Autodesk Inventor part; units mm, degrees
ref_plane "YZ Plane" through (0, 0, 0) normal (1, 0, 0) x (0, 1, 0)
ref_plane "XZ Plane" through (0, 0, 0) normal (0, 1, 0) x (-1, 0, 0)
ref_plane "XY Plane" through (0, 0, 0) normal (0, 0, 1) x (1, 0, 0)
sketch "Sketch1" plane through (0, 0, 0) normal (0, 1, 0) x (-1, 0, 0)
  circle A0 centre (0, 0) radius 3.81
  circle A1 centre (0, 0) radius 16.51
  line L0 (-7.4994, -5) -> (-1.1494, -5)
  line L1 (-1.1494, -5) -> (-1.1494, -11.35)
  line L2 (-1.1494, -11.35) -> (-7.4994, -11.35)
  line L3 (-7.4994, -11.35) -> (-7.4994, -5)
  line L4 (-7.4994, 5) -> (-1.1494, 5)
  line L5 (-1.1494, 5) -> (-1.1494, 11.35)
  line L6 (-1.1494, 11.35) -> (-7.4994, 11.35)
  line L7 (-7.4994, 11.35) -> (-7.4994, 5)
  circle A2 centre (-4.3244, -7.3812) radius 1.7526
  circle A3 centre (-4.3244, 7.3812) radius 1.7526
  line L8 (0, 0) -> (-10.16, 0)
  line L9 (0, 0) -> (10.16, 0)
  circle A4 centre (-10.16, 0) radius 1.7526
  circle A5 centre (10.16, 0) radius 1.7526
  line L10 (-4.3244, -8.175) -> (-10.16, 0)
  line L11 (-10.16, 0) -> (-4.3244, 8.175)
  line L12 (0, 0) -> (-7.2422, 4.0875)
  line L13 (0, 0) -> (-7.2422, -4.0875)
  line L14 (-7.2422, -4.0875) -> (-14.378, -8.115)
  line L15 (-7.2422, 4.0875) -> (-14.378, 8.115)
  line L16 (0, 0) -> (11.6743, -11.6743)
  line L17 (0, 0) -> (16.51, 0) construction
  line L18 (0, 0) -> (11.6743, 11.6743)
  line L19 (0, 0) -> (16.51, 0) construction
  line L20 (0, 0) -> (16.51, -6.8387)
  line L21 (0, 0) -> (17.8703, 0) construction
  line L22 (1.062, 0) -> (16.6655, -6.4632)
  line L23 (0.7509, -0.7509) -> (16.3545, -7.2141)
  point P0 (-3.318, 1.8727)
  point P1 (2.6941, 2.6941)
  point P2 (2.6941, -2.6941)
  point P3 (-3.318, -1.8727)
  point P4 (3.3444, -1.8252)
  point P5 (15.0931, -6.6917)
  point P6 (15.4042, -5.9407)
  point P7 (3.6554, -1.0742)
  dimension "d0" = 7.62
  dimension "d1" = 33.02
  dimension "d2" = 6.35
  dimension "d3" = 6.35
  dimension "d4" = 6.35
  dimension "d5" = 6.35
  dimension "d6" = 3.5052
  dimension "d7" = 3.5052
  dimension "d8" = 10.16
  dimension "d9" = 10.16
  dimension "d10" = 3.5052
  dimension "d11" = 3.5052
  dimension "d12" = 45
  dimension "d13" = 45
  dimension "d25" = 22.5
  dimension "d26" = 0.4064
  dimension "d27" = 0.4064
extrude "Extrusion1" add sketch "Sketch1" along normal blind 7.5184 contours A0 L18 A1 L22 | A5 | A3 | L4 L7 L6 L5 | A0 L12 L15 A1 L18 | L22 A1 L20 A0 | A0 L8 A4 L11 L12 | L20 A1 L23 A0 | A0 L13 L10 A4 L8 | L11 A4 L10 L14 A1 L15 | A2 | L0 L1 L2 L3 | A0 L16 A1 L14 L13 | L23 A1 L16 A0 | A4 L10 L8 | L8 L11 A4 | L11 L10 A4
extrude "Extrusion2" cut sketch "Sketch1" along normal blind 6.2992 contours A3 | L4 L7 L6 L5 | A0 L12 L15 A1 L18 | A2 | L0 L1 L2 L3 | A0 L16 A1 L14 L13
hole "Hole1" at (-10.16, 0, 0) at (10.16, 0, 0) at (4.3244, 0, -7.3812) at (4.3244, 0, 7.3812) direction (0, 1, 0) diameter 3.81 end through all
extrude "Extrusion3" cut sketch "Sketch1" along normal blind 7.5184 contours L22 A1 L20 A0 | L20 A1 L23 A0
properties part number "tab4"
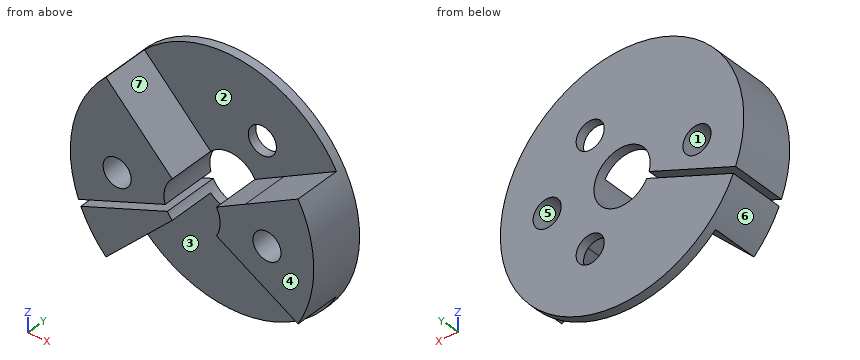
Design review of the part built by this model. Coordinates are the model's own, in mm. Face numbers are marked on the shaded views. A direction names the side the tool comes from. Give positions to 0.01 mm unless a question says otherwise; leave off trailing zeros. Order: outer loops, then holes, each group sorted by start corner. A loop starts at its lowest first (then second) coordinate and runs counter-clockwise, first axis right, second up. Notation, with made-up numbers: (6.25, 3.25) -> (43.25, 3.25) arc R17 ccw to (43.25, 18.25) -> close; hole circle Ø2 at (59.25, 54.5). An arc over 180 degrees is marked (long way). Write each question's results on one line, items separated by ' | '. Start each with the question number.
Q1. Wall thickness on L1, parallel to X at y = 5, z = 0 (3 decimals); L2, parallel to X at y = 3, z = -3.5; L3, parallel to Z at x = -11, y = 5: over which ranges is each line inside the solid? List them lowest first. Write a range as from..to.
Q2. Machinability: for the marked faces 1, 2 and 3, which of the approach directions +Z, -Z, +X, -X, +Y, -Y give a long, thin tool a straight path to every point of the face, cutting with its end or side? Answer none if there is none.
Q3. Add section C-C on z = 0. Give the boundary of the cut face in (x, y) (3 decimals), and give its area (3 significant figures).
Q4. For pin 1 (3 mm diameter, centred on x = 10.16, z = 0, fed in from -Y); pin 2 (1.5 mm diameter, centred on x = 8, y = 1, fed in from -Z); pin 3 (7.5 mm diameter, centred on x = 4, z = 12, fed in from -Y); pin 4 (6 mm diameter, centred on x = 11.5, z = 7, fed in from -Y), all flat-tipped, find the tip position at first contact; note any pin that passes through.
Q5. Mouldability with a two-part tool opening along X and no side actions: class the marked faces 4, 5, 6 and 7 as +X half, -X half, draft (parallel to the pull), parting line (faces both ways), or undercut.
Q6. Add section D-D on x = -11. Give the boundary of the cut face in (y, z).
Q7. Add section A-A on y = 3.25. Give the boundary of the cut face in (x, z) (1 decimal), and give its area (3 significant figures).
Q8. Add section B-B on x = 0. Give the boundary of the cut face in (y, z), and give its area (3 significant figures).
Found:
1) L1: x = -16.51..-12.065, -8.255..-3.81, 3.81..8.255, 12.065..16.51 | L2: x = -16.13..-9.51, -7.39..-3.5, 6.2..16.13 | L3: z = -11..-5, -4.12..-1.71, 1.71..11
2) face 1: +Y, -Y | face 2: +Z, -Y | face 3: -Z, -Y
3) outline: (-16.51, 0) -> (-12.065, 0) -> (-12.065, 7.518) -> (-16.51, 7.518) -> close; (-8.255, 0) -> (-3.81, 0) -> (-3.81, 7.518) -> (-8.255, 7.518) -> close; (3.81, 0) -> (8.255, 0) -> (8.255, 7.518) -> (3.81, 7.518) -> close; (12.065, 0) -> (16.51, 0) -> (16.51, 7.518) -> (12.065, 7.518) -> close | area: 134 mm2
4) pin 1: passes through | pin 2: stops at z = -4.94 | pin 3: stops at y = 6.3 | pin 4: stops at y = 0
5) face 4: draft | face 5: undercut | face 6: parting line | face 7: undercut
6) outline: (0, -11) -> (6.3, -11) -> (6.3, -12.31) -> (7.52, -12.31) -> (7.52, -5) -> (0, -5) -> close; (0, -4.12) -> (7.52, -4.12) -> (7.52, -1.71) -> (0, -1.71) -> close; (0, 1.71) -> (7.52, 1.71) -> (7.52, 12.31) -> (6.3, 12.31) -> (6.3, 11) -> (0, 11) -> close
7) outline: (-15.4, -5.9) -> (-3.7, -1.1) arc R3.8 cw to (-2.7, 2.7) -> (-11.7, 11.7) arc R16.5 ccw to start; (-15.1, -6.7) arc R16.5 ccw to (-11.7, -11.7) -> (-2.7, -2.7) arc R3.8 cw to (-3.3, -1.8) -> close; (3.3, -1.9) -> (7.2, -4.1) -> (14.4, -8.1) arc R16.5 ccw to (14.4, 8.1) -> (7.2, 4.1) -> (3.3, 1.9) arc R3.8 cw to start; hole circle Ø3.8 at (-10.2, 0); hole circle Ø3.8 at (10.2, 0) | area: 302 mm2
8) outline: (6.3, -16.51) -> (7.52, -16.51) -> (7.52, -3.81) -> (6.3, -3.81) -> close; (6.3, 3.81) -> (7.52, 3.81) -> (7.52, 16.51) -> (6.3, 16.51) -> close | area: 31.0 mm2
